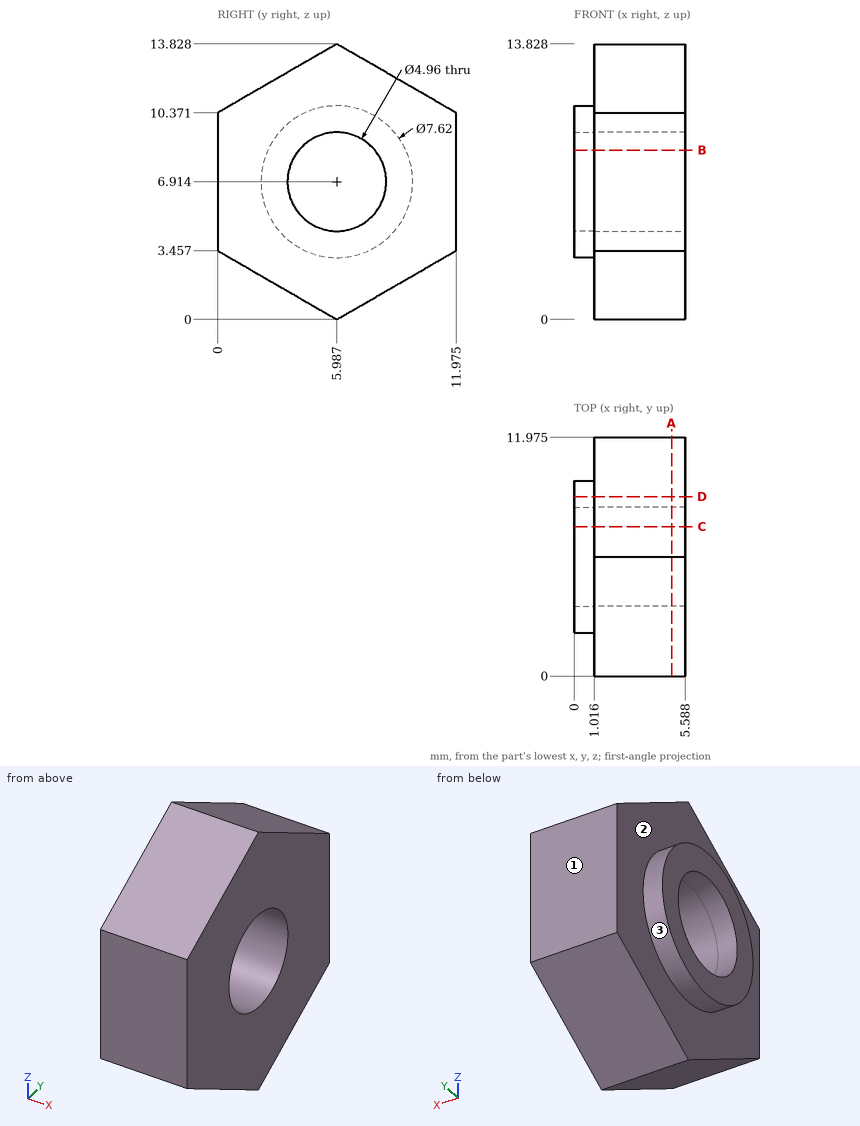
Job drawing, mm, ordinate dimensions from the low corner. One solid piece. Round coordinates to 2 decimals unless told otherwise and drop trailing zeros. Loops run counter-clockwise (first coordinate to the right, second up) from the corner with the lowest first, then second, coordinate; pieces in that order, holes last.
(1) Cut at A-A (x = 4.9). Give the cut face in (y, z) (1 decimal).
(2) Cut at B-B (z = 8.5). Give the cut face in (x, y) (1 decimal).
(3) Drop a flat-ended pin along its axis: pin 1 (3 mm diameter, centred on x = 3, z = 8.5, fed in from -Y). Give the stop position or say it passes through.
(4) Cut at D-D (y = 9). Give the cut face in (x, z) (1 decimal).
(5) Wall check: line 1 along X through (y, z) = (2.5, 3.5) (1 decimal); line 2 along Z through (x, y) = (1.6, 6) (1 decimal); line 3 along Z through (x, y) = (4.95, 6.75) (1 decimal). Give the ranges that are in metal, low to high.
(6) Two-plate mould, pull along Y, no slides. Class the marked faces 1, 2 and 3: +Y half, -Y half, draft (parallel to the pull), parting line (faces both ways), or undercut.
(7) Cut at C-C (y = 7.5). Give the cut face in (x, z) (1 decimal).
Findings below:
1. outline: (0, 3.5) - (6, 0) - (12, 3.5) - (12, 10.4) - (6, 13.8) - (0, 10.4) - close; hole circle Ø5 at (6, 6.9)
2. outline: (0, 2.5) - (1, 2.5) - (1, 0) - (5.6, 0) - (5.6, 4.1) - (0, 4.1) - close; (0, 7.9) - (5.6, 7.9) - (5.6, 12) - (1, 12) - (1, 9.5) - (0, 9.5) - close
3. pin 1: stops at y = 0
4. outline: (0, 4.6) - (1, 4.6) - (1, 1.7) - (5.6, 1.7) - (5.6, 12.1) - (1, 12.1) - (1, 9.2) - (0, 9.2) - close
5. line 1: x = 1 to 5.6
5. line 2: z = 0 to 4.4, 9.4 to 13.8
5. line 3: z = 0.4 to 4.6, 9.3 to 13.4
6. face 1: +Y half
6. face 2: draft
6. face 3: parting line
7. outline: (0, 3.4) - (1, 3.4) - (1, 0.9) - (5.6, 0.9) - (5.6, 4.9) - (0, 4.9) - close; (0, 8.9) - (5.6, 8.9) - (5.6, 13) - (1, 13) - (1, 10.4) - (0, 10.4) - close
